Geometry: final body of the model. Coordinates: model frame, mm. Face numbers are marked on the shaded views. A direction names the side the tool comes from. Give positions to 0.01 mm unless a question says otherwise; leave off trailing zeros.
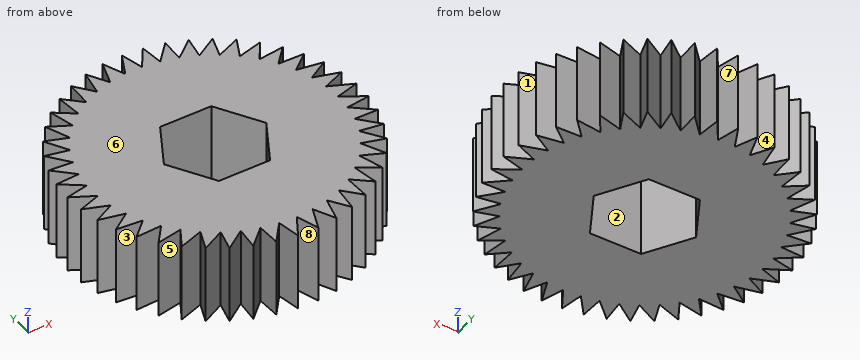
```python
from build123d import *

# Parameters (mm, degrees)
SCHIZZO1_R                   = 34.641016151
ESTRUSIONE_ESTRUSIONE1_DEPTH = 7.5
TAGLIO_ESTRUSIONE1_DEPTH     = 52.23475383
RIPETIZIONECIRCOLARE1_COUNT  = 45


with BuildPart() as part:
    # Schizzo1 → Estrusione-Estrusione1 (new, symmetric)
    with BuildSketch(Plane.XY):
        Circle(SCHIZZO1_R)
        Polygon((10, 0), (5, 8.660254038), (-5, 8.660254038), (-10, 0), (-5, -8.660254038), (5, -8.660254038), align=None, mode=Mode.SUBTRACT)
    extrude(amount=ESTRUSIONE_ESTRUSIONE1_DEPTH, both=True)

    # Schizzo2 → Taglio-Estrusione1 (cut, through all)
    with BuildSketch(Plane.XY.offset(7.5)):
        Polygon((-6.551263351, 35.534227752), (-1.911546114, 23.580132753), (5.348246738, 37.826793916), align=None)
    taglio_estrusione1 = extrude(amount=-TAGLIO_ESTRUSIONE1_DEPTH, mode=Mode.SUBTRACT)

    # RipetizioneCircolare1: Taglio-Estrusione1 ×45 about axis
    ripetizionecircolare1_axis = Axis((0, 0, 0), (0, 0, 1))
    for i in range(1, RIPETIZIONECIRCOLARE1_COUNT):
        add(taglio_estrusione1.rotate(ripetizionecircolare1_axis, i * 360 / RIPETIZIONECIRCOLARE1_COUNT), mode=Mode.SUBTRACT)


solid = part.part
```
Item 1: Line query: L1, parallel to Y at x = -18.5, z = -2.5; L2, parallel to X at y = -25, z = 3; L3, parallel to Y at x = -7, z = -4.75. Output: solid intervals per line, ascending.
Found:
L1: y = -19.49 to -17.86, -16.24 to 17.87
L2: x = -9.77 to -8.62, -6.22 to -4.28, -2.78 to -0.55, 0.68 to 2.87, 4.31 to 6.15, 8.3 to 9.43
L3: y = -23.49 to -5.2, 5.2 to 26.35
Item 2: Reachability of the marked faces 1, 2, 3 and 4 from +Z, -Z, +X, -X, +Y, -Y: full face, straight path, thin tool, end or side. Return the list, or none.
Found:
face 1: +Z, -Z, +X
face 2: +Z, -Z
face 3: +Z, -Z, -X
face 4: +Z, -Z, +Y
Item 3: Pin query (flat end, axial travel): pin 1 Ø2 at (y, z) = (-20.5, 0.5) entering from -X; pin 2 Ø1 at (x, z) = (-12, -4) entering from -Y; pin 3 Ø1 at (x, z) = (-13.5, 0.5) entering from +Y. Return the tip coordinate at first contact, or that it passes through.
Found:
pin 1: stops at x = -19.72
pin 2: stops at y = -23.9
pin 3: stops at y = 23.41
Item 4: Pull-direction query (Y, two-part tool) for the marked faces 5, 6, 7 and 8; classes: +Y half, -Y half, draft (parallel to the pull), parting line (faces both ways), or undercut.
Found:
face 5: undercut
face 6: draft
face 7: +Y half
face 8: -Y half
